from build123d import *

# Parameters (mm, degrees)
SKETCH1_R               = 5
BOSS_EXTRUDE1_DEPTH     = 5
SKETCH3_R               = 9
BOSS_EXTRUDE2_DEPTH     = 5
SKETCH2_R               = 2.5
CUT_EXTRUDE1_DEPTH      = 7
CUT_EXTRUDE1_DEPTH_BACK = 15


with BuildPart() as part:
    # Sketch1 → Boss-Extrude1 (new body)
    with BuildSketch(Plane(origin=(0, 0, 0), x_dir=(1, 0, 0), z_dir=(0, 1, 0))):
        Circle(SKETCH1_R)
    boss_extrude1 = extrude(amount=BOSS_EXTRUDE1_DEPTH)

    # Sketch3 → Boss-Extrude2 (add)
    with BuildSketch(Plane(origin=(0, 5, 0), x_dir=(1, 0, 0), z_dir=(0, 1, 0))):
        Circle(SKETCH3_R)
    boss_extrude2 = extrude(amount=BOSS_EXTRUDE2_DEPTH)

    # Mirror1: Boss-Extrude1, Boss-Extrude2 across plane
    add(boss_extrude1.mirror(Plane.ZX))
    add(boss_extrude2.mirror(Plane.ZX))

    # Sketch2 → Cut-Extrude1 (cut, two sides)
    with BuildSketch(Plane(origin=(0, 4, 0), x_dir=(1, 0, 0), z_dir=(0, 1, 0))) as cut_extrude1_sk:
        Circle(SKETCH2_R)
    extrude(amount=CUT_EXTRUDE1_DEPTH, mode=Mode.SUBTRACT)
    extrude(cut_extrude1_sk.sketch, amount=-CUT_EXTRUDE1_DEPTH_BACK, mode=Mode.SUBTRACT)


solid = part.part
Source: CAD feature listing. Evaluate the final solid. Frame: model axes, mm. A direction names the side the tool comes from. Give positions to 0.01 mm unless a question says otherwise; leave off trailing zeros. Write each loop counter-clockwise with the first axis right and the second up, starting at its lowest first coordinate (ties: lowest second). Pieces come first, ordered by that corner, then holes. Notation, with made-up numbers: M 55.5,77.5 L 109.5,77.5 A20 ccw 109.5,93.5 Z; hole C 12.5,18.25 d7. An arc over 180 degrees is marked long. Return JSON: item names as keys, results as strings. Group by question number.
1) Set-up query: faces 1 (the face through (4, -5, 4)), 2 (the face through (-1.172, -7.465, -8.923)). Return all of +Z, -Z, +X, -X, +Y, -Y with unobstructed straight access to the full face (end or side cutting, diameter ignored); none if empty.
2) Cut plane C-C, the plane y = -6. Output: boundary loops of the cut face in (x, z).
3) First-contact query: pin 1 Ø8 at (x, y) = (0, 0.5) entering from +Z; pin 2 Ø3 at (y, z) = (2, -3.5) entering from +X; pin 3 Ø2 at (y, z) = (7.5, -2.5) entering from +X. Flat tips, straight axial feed; report the tip coordinate or a pass-through.
4) Cut plane A-A, the plane x = 0. Output: boundary loops of the cut face in (y, z), then the cut area to 3 significant figures.
5) Cut plane B-B, the plane z = 0. Output: boundary loops of the cut face in (x, y).
6) Draft query along Y for faces 3 (the face through (-1.08, 0.07, 4.88)), 4 (the face through (4, 5, 4)), 5 (the face through (2, 10, 2)), 6 (the face through (-0.54, 0.14, 2.44)). Return one class per face: released by +Y, released by -Y, zero draft, split by the parting line, or undercut.
7) Ray query, L1, parallel to X at y = 2.5, z = 0; L2, parallel to Y at x = 2.5, z = -6.25. Return the intervals inside material, ascending.
8) Cut plane D-D, the plane x = -3.75. Output: boundary loops of the cut face in (y, z), then the cut area to 3 significant figures.
Data:
{
 "1": {"face 1": "none", "face 2": "+Y, -Y"},
 "2": {"outline": "C 0,0 d18; hole C 0,0 d5"},
 "3": {"pin 1": "stops at z = 5", "pin 2": "stops at x = 4.58", "pin 3": "stops at x = 8.87"},
 "4": {"outline": "M -10,-9 L -5,-9 L -5,-5 L 5,-5 L 5,-9 L 10,-9 L 10,-2.5 L -10,-2.5 Z; M -10,2.5 L 10,2.5 L 10,9 L 5,9 L 5,5 L -5,5 L -5,9 L -10,9 Z", "area": "180 mm²"},
 "5": {"outline": "M -9,-10 L -2.5,-10 L -2.5,10 L -9,10 L -9,5 L -5,5 L -5,-5 L -9,-5 Z; M 2.5,-10 L 9,-10 L 9,-5 L 5,-5 L 5,5 L 9,5 L 9,10 L 2.5,10 Z"},
 "6": {"face 3": "undercut", "face 4": "undercut", "face 5": "released by +Y", "face 6": "zero draft"},
 "7": {"L1": "x = -5 to -2.5, 2.5 to 5", "L2": "y = -10 to -5, 5 to 10"},
 "8": {"outline": "M -10,-8.18 L -5,-8.18 L -5,-3.31 L 5,-3.31 L 5,-8.18 L 10,-8.18 L 10,8.18 L 5,8.18 L 5,3.31 L -5,3.31 L -5,8.18 L -10,8.18 Z", "area": "230 mm²"}
}
